Source: CAD feature listing. Evaluate the final solid. Frame: model axes, mm. A direction names the side the tool comes from. Round coordinates to 2 decimals unless told otherwise and drop trailing zeros. Write each loop counter-clockwise with the first axis right and the second up, starting at its lowest first coordinate (ties: lowest second). Pieces come first, ordered by that corner, then holes. Notation, with made-up numbers: M -16.5,42 L 10.5,42 A23 ccw 10.5,68 Z; hole C 49,30.5 d6. An arc over 180 degrees is marked long. Use a Markdown table: item, result.
```python
from build123d import *

# Parameters (mm, degrees)
F0_R          = 49
F0_R_2        = 2.5
F1_DEPTH      = 6.7
F1_DEPTH_BACK = 7
F2_R          = 57.85
F2_R_2        = 55.35
F3_DEPTH      = 3
F4_R          = 14.9
F5_DEPTH      = 6.65
F7_DEPTH      = 30.3
F8_R          = 57.307814
F8_R_2        = 23.25
F9_DEPTH      = 6.25


with BuildPart() as f1:
    # F0 (on Front) → F1 (new body, two sides)
    with BuildSketch(Plane.XZ) as f1_sk:
        Circle(F0_R)
        with Locations((-21.5, -37.239092)):
            Circle(F0_R_2, mode=Mode.SUBTRACT)
        with BuildLine():
            ThreePointArc((2.041061, 4.902058), (3.356125, 4.114915), (4.391594, 2.984962))
            ThreePointArc((4.391594, 2.984962), (5.31, 0.000354), (4.391992, -2.984377))
            ThreePointArc((4.391992, -2.984377), (3.469883, -4.019454), (2.311288, -4.780591))
            Line((2.311288, -4.780591), (1.24348, -12.010569))
            ThreePointArc((1.24348, -12.010569), (-2.194471, -14.838607), (-4.660959, -11.132702))
            Line((-4.660959, -11.132702), (-3.683832, -4.516713))
            Line((-3.683832, -4.516713), (-3.594051, -3.908823))
            ThreePointArc((-3.594051, -3.908823), (-5.088714, -1.516936), (-5.147666, 1.302933))
            ThreePointArc((-5.147666, 1.302933), (-4.635012, 2.5909), (-3.806465, 3.702286))
            Line((-3.806465, 3.702286), (-5.274612, 10.855416))
            ThreePointArc((-5.274612, 10.855416), (-3.018653, 14.693117), (0.571674, 12.061227))
            Line((0.571674, 12.061227), (2.041061, 4.902058))
        make_face(mode=Mode.SUBTRACT)
        with Locations((43, 0)):
            Circle(F0_R_2, mode=Mode.SUBTRACT)
        with Locations((-21.5, 37.239092)):
            Circle(F0_R_2, mode=Mode.SUBTRACT)
    extrude(amount=F1_DEPTH)
    extrude(f1_sk.sketch, amount=-F1_DEPTH_BACK)

    # F2 (on face) → F3 (cut)
    with BuildSketch(Plane(origin=(0, 7, 0), x_dir=(-1, 0, 0), z_dir=(0, 1, 0))):
        Circle(F2_R)
        Circle(F2_R_2, mode=Mode.SUBTRACT)
    extrude(amount=-F3_DEPTH, mode=Mode.SUBTRACT)

    # F4 (on face) → F5 (cut)
    with BuildSketch(Plane.XZ.offset(6.7)):
        Circle(F4_R)
    extrude(amount=-F5_DEPTH, mode=Mode.SUBTRACT)

    # F6 (on face) → F7 (cut)
    with BuildSketch(Plane(origin=(0, 7, 0), x_dir=(-1, 0, 0), z_dir=(0, 1, 0))):
        with BuildLine():
            ThreePointArc((-49, 0), (-48.194169, 3.003433), (-45.99313, 5.200113))
            ThreePointArc((-45.99313, 5.200113), (-45.334188, 5.527347), (-44.64015, 5.771474))
            Line((-44.64015, 5.771474), (-24.327876, 11.667113))
            ThreePointArc((-24.327876, 11.667113), (-13.483488, 23.348029), (2.059675, 26.877142))
            Line((2.059675, 26.877142), (17.096325, 41.31434))
            ThreePointArc((17.096325, 41.31434), (17.755977, 41.92762), (18.5, 42.435245))
            ThreePointArc((18.5, 42.435245), (21.5, 43.239092), (24.5, 42.435245))
            ThreePointArc((24.5, 42.435245), (-24.5, 42.435245), (-49, 0))
        make_face()
        with BuildLine():
            ThreePointArc((49, 0), (42.435245, 24.5), (24.5, 42.435245))
            ThreePointArc((24.5, 42.435245), (26.746667, 40.149845), (27.496495, 37.034027))
            ThreePointArc((27.496495, 37.034027), (27.464398, 36.586443), (27.398941, 36.14251))
            ThreePointArc((27.398941, 36.14251), (27.327257, 35.809732), (27.236816, 35.481554))
            Line((27.236816, 35.481554), (22.268012, 15.224597))
            ThreePointArc((22.268012, 15.224597), (26.999999, -0.036464), (22.276739, -15.300227))
            Line((22.276739, -15.300227), (27.300915, -35.706322))
            ThreePointArc((27.300915, -35.706322), (27.435943, -36.364689), (27.496495, -37.034027))
            ThreePointArc((27.496495, -37.034027), (26.746667, -40.149845), (24.5, -42.435245))
            ThreePointArc((24.5, -42.435245), (42.435245, -24.5), (49, 0))
        make_face()
        with BuildLine():
            ThreePointArc((-45.818674, -5.296704), (-48.143542, -3.089333), (-49, 0))
            ThreePointArc((-49, 0), (-24.5, -42.435245), (24.5, -42.435245))
            ThreePointArc((24.5, -42.435245), (21.499855, -43.239092), (18.499749, -42.4351))
            ThreePointArc((18.499749, -42.4351), (17.89788, -42.037502), (17.348075, -41.570549))
            Line((17.348075, -41.570549), (2.111401, -26.9615))
            ThreePointArc((2.111401, -26.9615), (-13.509794, -23.421212), (-24.376516, -11.653896))
            Line((-24.376516, -11.653896), (-44.293281, -5.858961))
            ThreePointArc((-44.293281, -5.858961), (-45.075108, -5.629736), (-45.818674, -5.296704))
        make_face()
    extrude(amount=-F7_DEPTH, mode=Mode.SUBTRACT)

    # F8 (on face) → F9 (cut)
    with BuildSketch(Plane(origin=(0, 7, 0), x_dir=(-1, 0, 0), z_dir=(0, 1, 0))):
        Circle(F8_R)
        Circle(F8_R_2, mode=Mode.SUBTRACT)
    extrude(amount=-F9_DEPTH, mode=Mode.SUBTRACT)


solid = f1.part
```
Q1. Line query: L1, parallel to Z at x = -21.5, y = -4.25; L2, parallel to X at y = -4, z = 0; L3, parallel to Z at x = -0.5, y = -4.75. Output: solid intervals per line, ascending.
Results are:
| item | result |
|---|---|
| L1 | -43.24 to -39.74, -34.74 to 34.74, 39.74 to 43.24 |
| L2 | -27 to -14.9, 14.9 to 40.5, 45.5 to 49 |
| L3 | -27.04 to -14.89, 14.89 to 26.95 |
Q2. First-contact query: pin 1 Ø8 at (y, z) = (4.5, -17.5) entering from +X; pin 2 Ø5 at (x, z) = (-2.41, 11.75) entering from +Y; pin 3 Ø24 at (x, z) = (0, 0) entering from -Y; pin 4 Ø6 at (x, y) = (9.5, -3) entering from -Z. Flat tips, straight axial feed; report the tip coordinate or a pass-through.
Results are:
| item | result |
|---|---|
| pin 1 | x = 21.7 |
| pin 2 | through |
| pin 3 | y = -0.05 |
| pin 4 | z = -26.25 |
Q3. Mould query, pull axis X, two halves, no side actions, for faces 1 (the flat face through (34.626, -2.923, 8.678)), 2 (the flat face through (-15.3, -6.7, 0.6)), 3 (the flat face through (-24.787, -2.923, 25.495)), 4 (the flat face through (-4.53, 3.43, 7.23)). Classes: +X half, -X half, draft (parallel to the pull), parting line (faces both ways), or undercut.
Results are:
| item | result |
|---|---|
| face 1 | +X half |
| face 2 | draft |
| face 3 | -X half |
| face 4 | undercut |
Q4. Reachability of faces 5 (the flat face through (1.785, 3.426, -8.345)), 6 (the flat face through (8, 0.75, -22)), 7 (the cylindrical face through (14.9, -3.4, 0.1)) from +Z, -Z, +X, -X, +Y, -Y: full face, straight path, thin tool, end or side. Return the list, or none.
Results are:
| item | result |
|---|---|
| face 5 | +Y, -Y |
| face 6 | +Y |
| face 7 | -Y |
Q5. Section C-C on x = -16. Return loops of the section in (y, z), plus the area to 3 significant figures.
Results are:
| item | result |
|---|---|
| outline | M -6.7,-40.28 L 0.75,-40.28 L 0.75,-16.87 L 7,-16.87 L 7,16.87 L 0.75,16.87 L 0.75,40.26 L -6.7,40.26 Z |
| area | 811 mm^2 |
Q6. Section B-B on y = 6. Return loops of the section in (x, z), plus the area to 3 significant figures.
Results are:
| item | result |
|---|---|
| outline | C 0,0 d46.5; hole M -5.27,10.86 L -3.81,3.7 A5.31 ccw -5.15,1.3 A5.31 ccw -3.59,-3.91 L -3.68,-4.52 L -4.66,-11.13 A3 ccw long 1.24,-12.01 L 2.31,-4.78 A5.31 ccw 4.39,-2.98 A5.31 ccw 4.39,2.98 A5.31 ccw 2.04,4.9 L 0.57,12.06 A3 ccw long Z |
| area | 1,500 mm^2 |
Q7. Section D-D on y = -5. Give the number of separate pieces and of enclosed holes in the cut face, plus the area to 3 significant figures.
Results are:
| item | result |
|---|---|
| separate pieces | 1 |
| enclosed holes | 4 |
| area | 2,580 mm^2 |
Q8. Section A-A on x = 42. Return loops of the section in (y, z).
Results are:
| item | result |
|---|---|
| outline | M -6.7,-6.53 L 0.75,-6.53 L 0.75,-2.29 L -6.7,-2.29 Z; M -6.7,2.29 L 0.75,2.29 L 0.75,6.54 L -6.7,6.54 Z |
